```python
from build123d import *

# Parameters (mm, degrees)
BOSS_EXTRU_2_DEPTH      = 6
ENL_V_MAT_EXTRU_2_DEPTH = 10


with BuildPart() as part:
    # Esquisse1 → Boss.-Extru.2 (new body)
    with BuildSketch(Plane.XY):
        Polygon((-83.455959888, 54.712062767), (39.812904953, 35.321710103), (-38.614065462, -61.737082013), align=None)
        Polygon((28.614490816, 31.009457699), (-36.749378522, -49.882844686), (-74.12223269, 47.170077843), align=None, mode=Mode.SUBTRACT)
    extrude(amount=BOSS_EXTRU_2_DEPTH)

    # Esquisse2 → Enlèv. mat.-Extru.2 (cut)
    with BuildSketch(Plane.XY.offset(6)):
        Polygon((-24.872050824, -37.598295416), (19.142614995, 16.832478902), (21.475362465, 14.946136081), (-22.539303353, -39.484638237), align=None)
        Polygon((-57.172566376, 45.990983286), (11.977902, 35.118415816), (12.443869177, 38.082007318), (-56.706599198, 48.954574788), align=None)
        Polygon((-47.127893484, -35.578319674), (-72.28905902, 29.74331341), (-69.48956046, 30.821649076), (-44.328394923, -34.499984009), align=None)
    extrude(amount=-ENL_V_MAT_EXTRU_2_DEPTH, mode=Mode.SUBTRACT)


solid = part.part
```
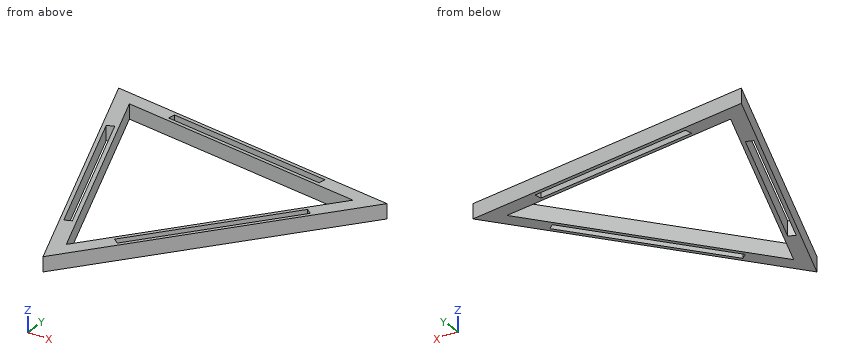
Check sheet for the modelled part. Datum: model origin and axes. Units: mm. Give positions to 0.01 mm unless a question says otherwise; leave off trailing zeros. Loops run counter-clockwise (first coordinate to the right, second up) from the corner with the lowest first, then second, coordinate; pieces in that order, holes last. Notation, with made-up numbers: M 87.25,-36.75 L 117.25,-36.75 A27 cw 117.25,-0.75 Z; hole C -28.5,-2 d2. An arc over 180 degrees is marked long. Answer as CSV lines item,"result".
Item 1: Sectioned sample at C-C, the plane x = 32. Enter the section's corners in (y, z).
Reply:
outline,"M 25.65,0 L 36.55,0 L 36.55,6 L 25.65,6 Z"
Item 2: Sectioned sample at B-B, the plane y = -8.5. Enter the section's corners in (x, z), then the cut area to 3 significant figures.
Reply:
outline,"M -59.11,0 L -57.56,0 L -57.56,6 L -59.11,6 Z; M -54.34,0 L -52.68,0 L -52.68,6 L -54.34,6 Z; M -3.31,0 L -1.34,0 L -1.34,6 L -3.31,6 Z; M 2.52,0 L 4.4,0 L 4.4,6 L 2.52,6 Z"
area,"42.4 mm^2"
Item 3: Scan lines: L1, parallel to Y at x = -11, z = 5.25; L2, parallel to X at y = 6, z = 5; L3, parallel to X at y = -7, z = 1. Record each from-to range of solid material in increasing order.
Reply:
L1,"-27.56 to -25.21, -20.44 to -18.02, 37.24 to 38.73, 41.77 to 43.31"
L2,"-64.7 to -63.14, -59.93 to -58.27, 8.41 to 10.38, 14.24 to 16.12"
L3,"-59.69 to -58.14, -54.92 to -53.26, -2.1 to -0.13, 3.73 to 5.62"
Item 4: Sectioned sample at A-A, the plane z = 4. Enter the section's corners in (x, y), then the cut area to 3 significant figures.
Reply:
outline,"M -83.46,54.71 L -38.61,-61.74 L 39.81,35.32 Z; hole M -74.12,47.17 L -36.75,-49.88 L 28.61,31.01 Z; hole M -72.29,29.74 L -47.13,-35.58 L -44.33,-34.5 L -69.49,30.82 Z; hole M -57.17,45.99 L 11.98,35.12 L 12.44,38.08 L -56.71,48.95 Z; hole M -24.87,-37.6 L -22.54,-39.48 L 21.48,14.95 L 19.14,16.83 Z"
area,"1,430 mm^2"
Item 5: Depth check by flat-ended pin: pin 1 Ø3 at (x, z) = (-10, 3.5) entering from +Y; pin 2 Ø2 at (x, z) = (24.5, 3) entering from +Y; pin 3 Ø3 at (x, z) = (-50, 4.5) entering from +Y. Enter the tip coordinate at first touch or a pass-through.
Reply:
pin 1,"y = 43.39"
pin 2,"y = 37.89"
pin 3,"y = 49.69"
